Geometry: final body of the model. Coordinates: model frame, mm. A direction names the side the tool comes from. Round coordinates to 2 decimals unless told otherwise and drop trailing zeros. Write each loop counter-clockwise with the first axis right and the second up, starting at its lowest first coordinate (ties: lowest second). Pieces come first, ordered by that corner, then holes. Notation, with made-up numbers: M 62,-20.75 L 95,-20.75 A21 cw 95,8.25 Z; hole C 4.25,-25.75 d3. An arc over 180 degrees is marked long. Use one line per item in the form item = value. Start each with the question number.
Item 1: Reachability of faces 3 (the flat face through (11, 21, 0)), 4 (the flat face through (10, 0, 3)), 5 (the cylindrical face through (-28.123, 0.41, -1.479)) from +Z, -Z, +X, -X, +Y, -Y: full face, straight path, thin tool, end or side. Return the list, or none.
Item 2: Ray query, probe 1 along Y at (x, z) = (-1, -1.5); probe 2 along Y at (x, z) = (-24, -2.5); probe 3 along X at (y, z) = (19, -1.25). Return the intervals inside material, ascending.
Item 3: Section query A-A (z = 2.75). Return loops of the section in (x, y), and give its area (3 significant figures).
Item 4: Pull-direction query (Y, two-part tool) for faces 1 (the flat face through (12, -13.8, -1)), 2 (the flat face through (0, -13.3, 3)); classes: pulls with the +Y half, pulls with the -Y half, needs draft (parallel to the pull), parting line crosses it, or undercut.
Item 5: Section query B-B (x = 0). State how many separate pieces and enclosed holes the cut face has, and give its area (3 significant figures).
Item 6: Pin query (flat end, axial travel): pin 1 Ø5 at (x, y) = (25, 0) entering from -Z; pin 2 Ø1.9 at (y, z) = (12, 2.5) entering from +X; pin 3 Ø5.5 at (x, y) = (-25, 0) entering from -Z. Return the tip coordinate at first contact, or that it passes through.
from build123d import *

# Parameters (mm, degrees)
SKETCH_1_R               = 17
EXTRUDE_1_DEPTH          = 5
SKETCH_2_R               = 30
SKETCH_2_R_2             = 17
EXTRUDE_2_DEPTH          = 2
EXTRUDE_START            = 3
SKETCH_3_R               = 30
SKETCH_3_R_2             = 20
EXTRUDE_3_DEPTH          = 3
CHAMFER_1_SIZE           = 2
PATTERN_CIRCULAR_1_COUNT = 8
SKETCH_6_R               = 4
CUT_EXTRUDE_1_DEPTH      = 2
SKETCH_7_R               = 2
CUT_EXTRUDE_2_DEPTH      = 43.720018727
PATTERN_CIRCULAR_2_COUNT = 4
CHAMFER_2_SIZE           = 0.5
CHAMFER_3_SIZE           = 3
SKETCH_8_W               = 27
SKETCH_8_H               = 3.3
CUT_EXTRUDE_3_DEPTH      = 43.720018727


with BuildPart() as part:
    # 草图1 → 凸台-拉伸1 (new body)
    with BuildSketch(Plane.XY):
        Circle(SKETCH_1_R)
        with BuildLine():
            ThreePointArc((-10, 9), (-10.707106781, 10.707106781), (-9, 10))
            Line((-9, 10), (-7.15, 10))
            Line((-7.15, 10), (-7.15, 13.3))
            Line((-7.15, 13.3), (7.15, 13.3))
            Line((7.15, 13.3), (7.15, 10))
            Line((7.15, 10), (9, 10))
            ThreePointArc((9, 10), (10, 11), (11, 10))
            ThreePointArc((11, 10), (10.707106781, 9.292893219), (10, 9))
            Line((10, 9), (10, -9))
            ThreePointArc((10, -9), (10.707106781, -9.292893219), (11, -10))
            ThreePointArc((11, -10), (10, -11), (9, -10))
            Line((9, -10), (7.15, -10))
            Line((7.15, -10), (7.15, -13.3))
            Line((7.15, -13.3), (-7.15, -13.3))
            Line((-7.15, -13.3), (-7.15, -10))
            Line((-7.15, -10), (-9, -10))
            ThreePointArc((-9, -10), (-10.707106781, -10.707106781), (-10, -9))
            Line((-10, -9), (-10, 9))
        make_face(mode=Mode.SUBTRACT)
    extrude(amount=EXTRUDE_1_DEPTH)

    # 草图2 → 凸台-拉伸2 (add)
    with BuildSketch(Plane(origin=(0, 0, 0), x_dir=(-1, 0, 0), z_dir=(0, 0, -1))):
        Circle(SKETCH_2_R)
        Circle(SKETCH_2_R_2, mode=Mode.SUBTRACT)
    extrude(amount=-EXTRUDE_2_DEPTH)

    # 草图3 → 凸台-拉伸3 (add)
    with BuildSketch(Plane(origin=(0, 0, 0), x_dir=(-1, 0, 0), z_dir=(0, 0, -1)).offset(EXTRUDE_START)):
        Circle(SKETCH_3_R)
        Circle(SKETCH_3_R_2, mode=Mode.SUBTRACT)
    extrude(amount=-EXTRUDE_3_DEPTH)

    # 倒角1
    chamfer_1_edges = [part.edges().sort_by_distance(p)[0] for p in [
        (-17, 0, 2),
    ]]
    chamfer(chamfer_1_edges, length=CHAMFER_1_SIZE)

    # 草图5 → 切除-旋转1 (revolve, cut)
    with BuildSketch(Plane(origin=(0, 0, 0), x_dir=(0, 0, -1), z_dir=(1, 0, 0)), mode=Mode.PRIVATE) as cut_revolve_1_sk:
        with BuildLine():
            Line((-3.15, 25), (3.15, 25))
            Line((3.15, 25), (3.15, 28.15))
            Line((3.15, 28.15), (0, 28.15))
            ThreePointArc((0, 28.15), (-2.227386361, 27.227386361), (-3.15, 25))
        make_face()
    cut_revolve_1 = revolve(cut_revolve_1_sk.sketch.rotate(Axis((0, 25, 998.877863865), (0, 0, -1)), 270), axis=Axis((0, 25, 998.877863865), (0, 0, -1)), mode=Mode.SUBTRACT)

    # 阵列(圆周)1: 切除-旋转1 ×8 about axis
    pattern_circular_1_axis = Axis((0, 0, 0), (0, 0, 1))
    for i in range(1, PATTERN_CIRCULAR_1_COUNT):
        add(cut_revolve_1.rotate(pattern_circular_1_axis, i * 360 / PATTERN_CIRCULAR_1_COUNT), mode=Mode.SUBTRACT)

    # 草图6 → 切除-拉伸1 (cut)
    with BuildSketch(Plane.XY.offset(2)):
        with Locations((9.567085809, 23.096988313)):
            Circle(SKETCH_6_R)
    cut_extrude_1 = extrude(amount=-CUT_EXTRUDE_1_DEPTH, mode=Mode.SUBTRACT)

    # 草图7 → 切除-拉伸2 (cut, through all)
    with BuildSketch(Plane.XY):
        with Locations((9.567085809, 23.096988313)):
            Circle(SKETCH_7_R)
    cut_extrude_2 = extrude(amount=-CUT_EXTRUDE_2_DEPTH, mode=Mode.SUBTRACT)

    # 阵列(圆周)2: 切除-拉伸1, 切除-拉伸2 ×4 about axis
    pattern_circular_2_axis = Axis((0, 0, 0), (0, 0, 1))
    add([cut_extrude_1.rotate(pattern_circular_2_axis, i * 360 / PATTERN_CIRCULAR_2_COUNT) for i in range(1, PATTERN_CIRCULAR_2_COUNT)], mode=Mode.SUBTRACT)
    add([cut_extrude_2.rotate(pattern_circular_2_axis, i * 360 / PATTERN_CIRCULAR_2_COUNT) for i in range(1, PATTERN_CIRCULAR_2_COUNT)], mode=Mode.SUBTRACT)

    # 倒角2
    chamfer_2_edges = [part.edges().sort_by_distance(p)[0] for p in [
        (10, 0, 0),
        (8.075, 10, 0),
        (0, 13.3, 0),
        (-8.075, 10, 0),
        (-10, 0, 0),
        (-8.075, -10, 0),
        (0, -13.3, 0),
        (8.075, -10, 0),
    ]]
    chamfer(chamfer_2_edges, length=CHAMFER_2_SIZE)

    # 倒角3
    chamfer_3_edges = [part.edges().sort_by_distance(p)[0] for p in [
        (20, 0, 0),
    ]]
    chamfer(chamfer_3_edges, length=CHAMFER_3_SIZE - 0.0001)  # a hair under: the kernel refuses the full size

    # 草图8 → 切除-拉伸3 (cut, through all)
    with BuildSketch(Plane(origin=(0, 0, 0), x_dir=(-1, 0, 0), z_dir=(0, 0, -1))):
        with Locations((0, 12.15)):
            Rectangle(SKETCH_8_W, SKETCH_8_H)
        with Locations((0, -12.15)):
            Rectangle(SKETCH_8_W, SKETCH_8_H)
    extrude(amount=CUT_EXTRUDE_3_DEPTH, mode=Mode.SUBTRACT)


solid = part.part
Working result:
q1.face_3 = +Z
q1.face_4 = +Z, -Z
q1.face_5 = -Z
q2.probe_1 = -29.98 to -27.99, -22.01 to -18.47, 18.47 to 22.01, 27.99 to 29.98
q2.probe_2 = -18 to -2.99, 2.99 to 7.78, 11.35 to 18
q2.probe_3 = -23.22 to -20.54, -14.82 to 14.82, 20.54 to 23.22
q3.outline = C 0,0 d36.5; hole M -10,-9 A1 ccw long -9,-10 L -7.15,-10 L -7.15,-13.3 L 7.15,-13.3 L 7.15,-10 L 9,-10 A1 ccw long 10,-9 L 10,9 A1 ccw long 9,10 L 7.15,10 L 7.15,13.3 L -7.15,13.3 L -7.15,10 L -9,10 A1 ccw long -10,9 Z
q3.area = 543 mm²
q4.face_1 = undercut
q4.face_2 = undercut
q5.separate_pieces = 4
q5.enclosed_holes = 0
q5.area = 101 mm²
q6.pin_1 = 1.92
q6.pin_2 = 27.83
q6.pin_3 = 1.54
